Drawing for the job (mm, zero at the part's lowest x, y, z). A direction names the side the tool comes from. Coordinates: 2 decimals unless noted, no trailing zeros. Order: outer loops, then holes, each group sorted by start corner. A loop starts at its lowest first (then second) coordinate and runs counter-clockwise, first axis right, second up. Notation, with made-up numbers: M 12,-19 L 16,-19 A22 cw 16,8 Z; hole C 78,19.5 d10. An arc over 180 degrees is marked long. Write item = value, one per line. Start each with the question number.
Q1. Pin check, flat tips, straight feed: P1, Ø3, axis at x = 128, y = 12.5, coming from the -Z side; P2, Ø12, axis at x = 256, y = 27.5, coming from the +Z side; P3, Ø3, axis at y = 16, z = 16, coming from the +X side; P4, Ø8, axis at y = 17.5, z = 17, coming from the -X side. Stop position of each tip, or through.
Q2. Drill centre lines: probe 1 along Y at (x, z) = (255.97, 2.75); probe 2 along Z at (x, y) = (25, 33.5); probe 3 along X at (y, z) = (7, 16). Where is each one in solid material? Low to high.
Q3. Band-saw the part on C-C on z = 5.25. Write the cut outline in (x, y).
Q4. Band-saw the part on A-A on x = 20. Write the cut outline in (y, z).
Q5. Band-saw the part on B-B on y = 20. Write the cut outline in (x, z), plus the area to 3 significant figures.
Q6. Band-saw the part on D-D on y = 30. Write the cut outline in (x, z).
Q7. 3-axis set-ups, long thin cutter, end or side, ignore diameter. For the marked faces 1, 2 and 3: which of +Z, -Z, +X, -X, +Y, -Y reach the whole face in a straight line?
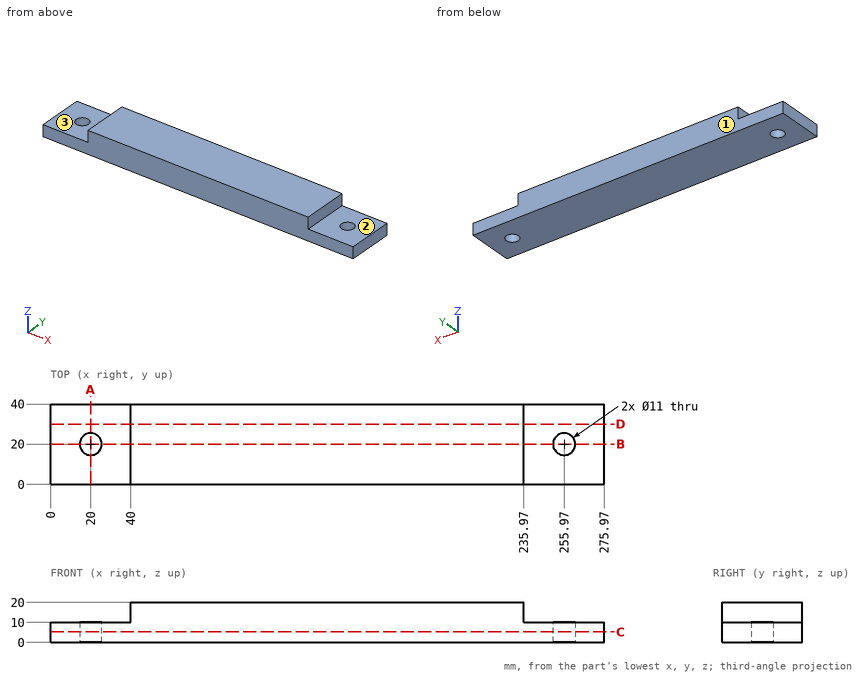
Recorded:
q1.P1 = 0
q1.P2 = 10
q1.P3 = 235.97
q1.P4 = 40
q2.probe_1 = 0 to 14.5, 25.5 to 40
q2.probe_2 = 0 to 10
q2.probe_3 = 40 to 235.97
q3.outline = M 0,0 L 275.97,0 L 275.97,40 L 0,40 Z; hole C 20,20 d11; hole C 255.97,20 d11
q4.outline = M 0,0 L 14.5,0 L 14.5,10 L 0,10 Z; M 25.5,0 L 40,0 L 40,10 L 25.5,10 Z
q5.outline = M 0,0 L 14.5,0 L 14.5,10 L 0,10 Z; M 25.5,0 L 250.47,0 L 250.47,10 L 235.97,10 L 235.97,20 L 40,20 L 40,10 L 25.5,10 Z; M 261.47,0 L 275.97,0 L 275.97,10 L 261.47,10 Z
q5.area = 4,500 mm2
q6.outline = M 0,0 L 275.97,0 L 275.97,10 L 235.97,10 L 235.97,20 L 40,20 L 40,10 L 0,10 Z
q7.face_1 = +Z, -Z, +X, -X, +Y
q7.face_2 = +Z, +X, +Y, -Y
q7.face_3 = +Z, -X, +Y, -Y
